Model file for the job. Use its own axes, mm. Face numbers are marked on the shaded views. A direction names the side the tool comes from. Coordinates: 2 decimals unless noted, no trailing zeros. Loops run counter-clockwise (first coordinate to the right, second up) from the corner with the lowest first, then second, coordinate; pieces in that order, holes last. Notation, with made-up numbers: (45, -19) - (92, -19) arc R29 cw to (92, 2) - close; hole circle Ø8 at (30.5, -7). An arc over 180 degrees is marked (long way). Write each question's results on one line, items separated by ' | '. Start each with the question number.
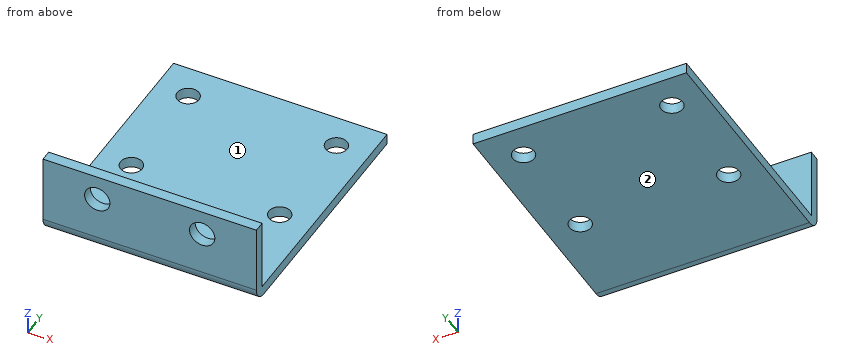
```python
from build123d import *

# Parameters (mm, degrees)
F0_W     = 59
F0_H     = 23.1
F0_R     = 3.5
F1_DEPTH = 1.5
F3_W     = 59
F3_H     = 66
F3_R     = 3
F4_DEPTH = 3
F5_R     = 4


with BuildPart() as f1:
    # F0 (on Front) → F1 (new body, symmetric)
    with BuildSketch(Plane.XZ):
        Rectangle(F0_W, F0_H)
        with Locations((-14.5, 4.55)):
            Circle(F0_R, mode=Mode.SUBTRACT)
        with Locations((14.5, 4.55)):
            Circle(F0_R, mode=Mode.SUBTRACT)
    extrude(amount=F1_DEPTH, both=True)

    # F3 (on offset) → F4 (join)
    with BuildSketch(Plane(origin=(0, 0, -11.55), x_dir=(1, 0, 0), z_dir=(0, 0, -1))):
        with Locations((0, -34.5)):
            Rectangle(F3_W, F3_H)
        with Locations((-20.5, -58)):
            Circle(F3_R, mode=Mode.SUBTRACT)
        with Locations((20.5, -58)):
            Circle(F3_R, mode=Mode.SUBTRACT)
        with Locations((-20.5, -28)):
            Circle(F3_R, mode=Mode.SUBTRACT)
        with Locations((20.5, -28)):
            Circle(F3_R, mode=Mode.SUBTRACT)
    extrude(amount=-F4_DEPTH)

    # F5
    f5_edges = [f1.edges().sort_by_distance(p)[0] for p in [
        (0, -1.5, -11.55),
    ]]
    fillet(f5_edges, radius=F5_R)


solid = f1.part
```
Q1. Pin check, flat tips, straight feed: pin 1 (17.5 mm diameter, centred on x = -14.5, y = 50, fed in from +Z); pin 2 (12 mm diameter, centred on y = 21, z = 2, fed in from +X) (1 decimal); pin 3 (1 mm diameter, centred on x = 21.5, z = 2.5, fed in from +Y). Stop position of each tip, or through.
Q2. Drill centre lines: L1, parallel to X at y = 58, z = -9.2; L2, parallel to Y at x = -3, z = 8.25; L3, parallel to Z at x = 19, y = 11. Where is each one in solid material? Low to high. Write a range as from..to.
Q3. Cut at B-B (y = 28). List the corners of the cut face in (x, z), and give its area (3 significant figures).
Q4. Which spindle directions (+Z, -Z, +X, -X, +Y, -Y) get a long thin tool onto all of the face, cutting with end or side? Do the marked faces 1 and 2. Say none if no direction does.
Q5. Cut at C-C (x = 20.5). List the corners of the cut face in (y, z).
Q6. Cut at D-D (z = 4.55). List the corners of the cut face in (x, y).
Q7. Cut at A-A (x = -14.5). List the corners of the cut face in (y, z).
Check result:
1) pin 1: z = -8.55 | pin 2: through | pin 3: y = 1.5
2) L1: -29.5..-23.5, -17.5..17.5, 23.5..29.5 | L2: -1.5..1.5 | L3: -11.55..-8.55
3) outline: (-29.5, -11.55) - (-23.5, -11.55) - (-23.5, -8.55) - (-29.5, -8.55) - close; (-17.5, -11.55) - (17.5, -11.55) - (17.5, -8.55) - (-17.5, -8.55) - close; (23.5, -11.55) - (29.5, -11.55) - (29.5, -8.55) - (23.5, -8.55) - close | area: 141 mm²
4) face 1: +Z, +X, -X, +Y | face 2: -Z, +X, -X, +Y, -Y
5) outline: (-1.5, -7.55) arc R4 ccw to (2.5, -11.55) - (25, -11.55) - (25, -8.55) - (1.5, -8.55) - (1.5, 11.55) - (-1.5, 11.55) - close; (31, -11.55) - (55, -11.55) - (55, -8.55) - (31, -8.55) - close; (61, -11.55) - (67.5, -11.55) - (67.5, -8.55) - (61, -8.55) - close
6) outline: (-29.5, -1.5) - (-18, -1.5) - (-18, 1.5) - (-29.5, 1.5) - close; (-11, -1.5) - (11, -1.5) - (11, 1.5) - (-11, 1.5) - close; (18, -1.5) - (29.5, -1.5) - (29.5, 1.5) - (18, 1.5) - close
7) outline: (-1.5, -7.55) arc R4 ccw to (2.5, -11.55) - (67.5, -11.55) - (67.5, -8.55) - (1.5, -8.55) - (1.5, 1.05) - (-1.5, 1.05) - close; (-1.5, 8.05) - (1.5, 8.05) - (1.5, 11.55) - (-1.5, 11.55) - close
